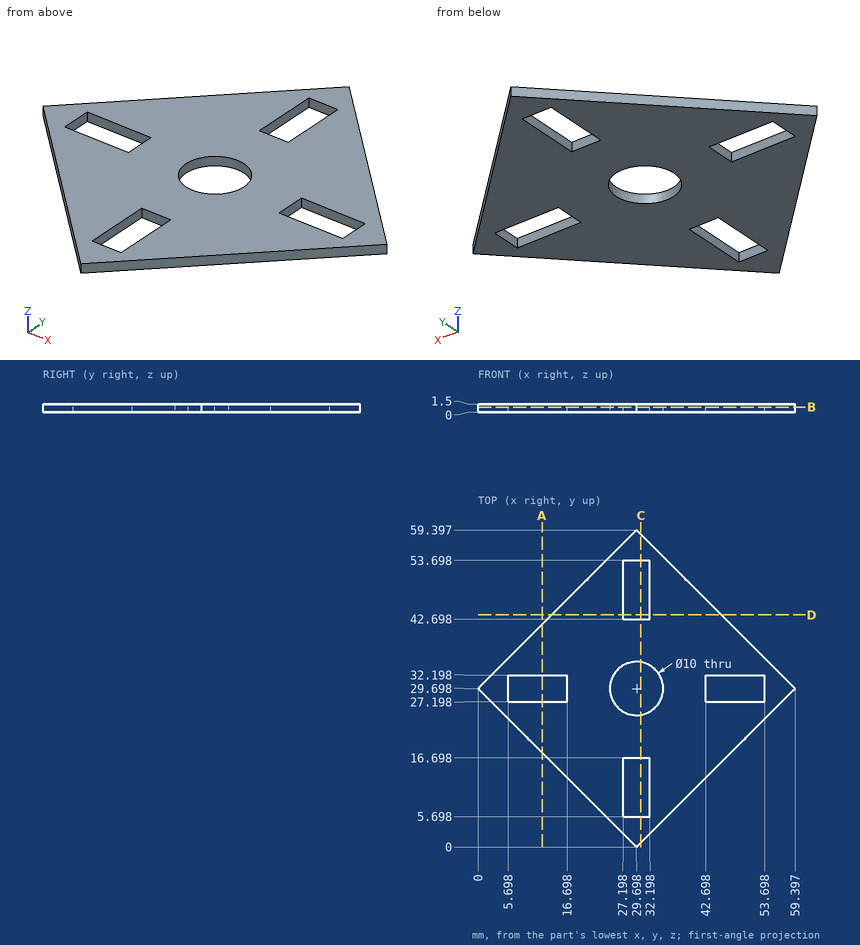
The drawing under review shows one solid part. Ordinate dimensions are in mm from its lowest x, y, z. Give positions to 0.01 mm unless a question says otherwise; leave off trailing zeros. Write each loop counter-clockwise with the first axis right and the second up, starting at its lowest first coordinate (ties: lowest second). Pieces come first, ordered by that corner, then holes. Notation, with made-up numbers: M 18.25,11 L 76.25,11 A29 cw 76.25,31 Z; hole C 51.25,-34 d4. An arc over 180 degrees is marked long. Write each question's results on one line, items separated by ' | '. Start each with the question number.
1. We need section C-C (x = 30.5). Write out the cut boundary in (y, z) (1 decimal).
2. We need section B-B (z = 0.9). Write out the cut boundary in (x, y).
3. Insertion check: pin 1 Ø4 at (x, y) = (44.5, 29.5) entering from -Z; pin 2 Ø0.8 at (x, z) = (13.5, 1) entering from -Y; pin 3 Ø9 at (x, y) = (29.7, 29.7) entering from -Z; pin 4 Ø0.8 at (x, z) = (11.5, 1) entering from +Y. Each pin has a flat end and moves straight along its axis. Give the tip position at first contact, or say it passes through.
4. We need section A-A (x = 12). Write out the cut boundary in (y, z), and give its area (3 significant figures).
5. For probe 1 along X at (y, z) = (13, 0.35); probe 2 along X at (y, z) = (8.5, 0.5); probe 3 along Y at (x, z) = (31, 1.2) (1 decimal), list the stretches that pass through material, from the lowest coordinate up. Write a range as [from, to].
6. We need section D-D (y = 43.5). Write out the cut boundary in (x, z) (1 decimal).
Results found:
1) outline: M 0.8,0 L 5.7,0 L 5.7,1.5 L 0.8,1.5 Z; M 16.7,0 L 24.8,0 L 24.8,1.5 L 16.7,1.5 Z; M 34.6,0 L 42.7,0 L 42.7,1.5 L 34.6,1.5 Z; M 53.7,0 L 58.6,0 L 58.6,1.5 L 53.7,1.5 Z
2) outline: M 0,29.7 L 29.7,0 L 59.4,29.7 L 29.7,59.4 Z; hole M 5.7,27.2 L 16.7,27.2 L 16.7,32.2 L 5.7,32.2 Z; hole C 29.7,29.7 d10; hole M 27.2,5.7 L 32.2,5.7 L 32.2,16.7 L 27.2,16.7 Z; hole M 27.2,42.7 L 32.2,42.7 L 32.2,53.7 L 27.2,53.7 Z; hole M 42.7,27.2 L 53.7,27.2 L 53.7,32.2 L 42.7,32.2 Z
3) pin 1: stops at z = 0 | pin 2: stops at y = 15.8 | pin 3: passes through | pin 4: stops at y = 41.6
4) outline: M 17.7,0 L 27.2,0 L 27.2,1.5 L 17.7,1.5 Z; M 32.2,0 L 41.7,0 L 41.7,1.5 L 32.2,1.5 Z | area: 28.5 mm^2
5) probe 1: x = [16.7, 27.2], [32.2, 42.7] | probe 2: x = [21.2, 27.2], [32.2, 38.2] | probe 3: y = [1.3, 5.7], [16.7, 24.9], [34.5, 42.7], [53.7, 58.1]
6) outline: M 13.8,0 L 27.2,0 L 27.2,1.5 L 13.8,1.5 Z; M 32.2,0 L 45.6,0 L 45.6,1.5 L 32.2,1.5 Z
